The model under review builds one solid part; all positions refer to its coordinate system, in mm. A direction names the side the tool comes from. Coordinates: 2 decimals unless noted, no trailing zeros. Loops run counter-clockwise (first coordinate to the right, second up) from the corner with the lowest first, then second, coordinate; pieces in that order, holes last. Notation, with made-up numbers: M 26,-3.75 L 61,-3.75 A3 cw 61,0.25 Z; hole C 85,2 d6. An arc over 180 degrees is marked long. Return JSON: item names as keys, results as strings.
```python
from build123d import *

# Parameters (mm, degrees)
SKETCH_1_R          = 2
EXTRUDE_1_DEPTH     = 2
SKETCH_2_R          = 0.75
CUT_EXTRUDE_1_DEPTH = 102.941600929
FILLET_1_R          = 2
SKETCH_3_W          = 5.7
SKETCH_3_H          = 27.500414906
CUT_EXTRUDE_2_DEPTH = 102.941600929
FILLET_2_R          = 1


with BuildPart() as part:
    # 草图1 → 凸台-拉伸1 (new body)
    with BuildSketch(Plane(origin=(0, 0, 0), x_dir=(1, 0, 0), z_dir=(0, 1, 0))):
        Polygon((7.5, 100), (7.5, -7.5), (-7.5, -7.5), (-17.7, 12), (-17.7, 22), (-19.7, 22), (-19.7, 42), (-17.7, 42), (-17.7, 57), (-19.7, 57), (-19.7, 77), (-17.7, 77), (-17.7, 87), (-7.5, 100), align=None)
        with Locations(Location((0, 25, 0), (0, 0, 270))):
            Circle(SKETCH_1_R, mode=Mode.SUBTRACT)
        with Locations(Location((0, 0, 0), (0, 0, 270))):
            Circle(SKETCH_1_R, mode=Mode.SUBTRACT)
        with Locations(Location((0, 72, 0), (0, 0, 270))):
            Circle(SKETCH_1_R, mode=Mode.SUBTRACT)
        with Locations(Location((0, 95, 0), (0, 0, 270))):
            Circle(SKETCH_1_R, mode=Mode.SUBTRACT)
    extrude(amount=EXTRUDE_1_DEPTH)

    # 草图2 → 切除-拉伸1 (cut, through all)
    with BuildSketch(Plane(origin=(0, 2, 0), x_dir=(1, 0, 0), z_dir=(0, 1, 0))):
        with Locations((-17.7, 77.75)):
            Circle(SKETCH_2_R)
        with Locations((-17.7, 56.25)):
            Circle(SKETCH_2_R)
        with Locations((-17.7, 42.75)):
            Circle(SKETCH_2_R)
        with Locations((-17.7, 21.25)):
            Circle(SKETCH_2_R)
    extrude(amount=-CUT_EXTRUDE_1_DEPTH, mode=Mode.SUBTRACT)

    # 圆角1
    fillet_1_edges = [part.edges().sort_by_distance(p)[0] for p in [
        (-17.7, 1, -87),
        (-7.5, 1, -100),
        (7.5, 1, -100),
        (7.5, 1, 7.5),
        (-7.5, 1, 7.5),
        (-17.7, 1, -12),
    ]]
    fillet(fillet_1_edges, radius=FILLET_1_R)

    # 草图3 → 切除-拉伸2 (cut, through all)
    with BuildSketch(Plane(origin=(0, 2, 0), x_dir=(1, 0, 0), z_dir=(0, 1, 0))):
        with BuildLine():
            Line((-4, 9), (-4, 16))
            ThreePointArc((-4, 16), (0, 20), (4, 16))
            Line((4, 16), (4, 9))
            ThreePointArc((4, 9), (0, 5), (-4, 9))
        make_face()
        with BuildLine():
            Line((4, 63), (4, 34))
            ThreePointArc((4, 34), (0, 30), (-4, 34))
            Line((-4, 34), (-4, 63))
            ThreePointArc((-4, 63), (0, 67), (4, 63))
        make_face()
        Polygon((-7.5, 92.710034389), (-13.2, 85.445328506), (-13.2, 65.209619483), (-7.5, 65.209619483), align=None)
        Polygon((-13.2, 13.105848495), (-7.5, 2.208789672), (-7.5, 29.709204577), (-13.2, 29.709204577), align=None)
        with Locations((-10.35, 47.45941203)):
            Rectangle(SKETCH_3_W, SKETCH_3_H)
    extrude(amount=-CUT_EXTRUDE_2_DEPTH, mode=Mode.SUBTRACT)

    # 圆角2
    fillet_2_edges = [part.edges().sort_by_distance(p)[0] for p in [
        (-7.5, 1, -92.710034389),
        (-7.5, 1, -65.209619483),
        (-13.2, 1, -65.209619483),
        (-13.2, 1, -85.445328506),
        (-7.5, 1, -29.709204577),
        (-7.5, 1, -2.208789672),
        (-13.2, 1, -13.105848495),
        (-13.2, 1, -29.709204577),
        (-13.2, 1, -33.709204577),
        (-13.2, 1, -61.209619483),
        (-7.5, 1, -61.209619483),
        (-7.5, 1, -33.709204577),
        (-19.7, 1, -22),
        (-19.7, 1, -42),
        (-19.7, 1, -57),
        (-19.7, 1, -77),
    ]]
    fillet(fillet_2_edges, radius=FILLET_2_R)


solid = part.part
```
1. Add section A-A on x = 0. Give the boundary of the cut face in (y, z), plus the area to 3 significant figures.
Check values:
{"outline": "M 0,-100 L 2,-100 L 2,-97 L 0,-97 Z; M 0,-93 L 2,-93 L 2,-74 L 0,-74 Z; M 0,-70 L 2,-70 L 2,-67 L 0,-67 Z; M 0,-30 L 2,-30 L 2,-27 L 0,-27 Z; M 0,-23 L 2,-23 L 2,-20 L 0,-20 Z; M 0,-5 L 2,-5 L 2,-2 L 0,-2 Z; M 0,2 L 2,2 L 2,7.5 L 0,7.5 Z", "area": "79.0 mm²"}
2. To check wall thickness, follow line 1 (X direction, y = 1.25, z = -25); line 2 (Z direction, x = -18.5, y = 0.6); line 3 (X direction, y = 1.8, z = -73). State the ranges of each line that lie inside material, in increasing order.
Check values:
{"line 1": "-19.7 to -13.2, -7.5 to -2, 2 to 7.5", "line 2": "-77 to -57, -42 to -22", "line 3": "-19.7 to -13.2, -7.5 to -1.73, 1.73 to 7.5"}
3. Add section C-C on z = -64. Give the boundary of the cut face in (x, y).
Check values:
{"outline": "M -19.7,0 L -3.87,0 L -3.87,2 L -19.7,2 Z; M 3.87,0 L 7.5,0 L 7.5,2 L 3.87,2 Z"}
4. Add section D-D on y = 0.8. State how many separate pieces and enclosed holes the cut face has, plus the area to 3 significant figures.
Check values:
{"separate pieces": "1", "enclosed holes": "9", "area": "1,770 mm²"}
5. Insertion check: pin 1 Ø0.6 at (x, y) = (-10, 1.5) entering from -Z; pin 2 Ø0.6 at (x, y) = (-9.5, 0.5) entering from +Z; pin 3 Ø5 at (x, z) = (0, -72) entering from -Y; pin 4 Ø1 at (y, z) = (1, -47) entering from -X. Each pin has a flat end and moves straight along its axis. Give the tip position at first contact, or say it passes through.
Check values:
{"pin 1": "z = -97.2", "pin 2": "z = 4.25", "pin 3": "y = 0", "pin 4": "x = -17.7"}
6. The part is to be moulded in two halves that separate along Z. For faces 1 (the face through (0, 1, -20)), 2 (the face through (-6, 2, -47)), 3 (the face through (-7.5, 1, -17)), 4 (the face through (6.93, 1.01, -99.4)), say which applies: released by +Z, released by -Z, zero draft, split by the parting line, or undercut.
Check values:
{"face 1": "undercut", "face 2": "zero draft", "face 3": "undercut", "face 4": "released by -Z"}
7. Machinability: for faces 5 (the face through (-12.7, 0.99, -2.44)), 6 (the face through (-11.11, 1.01, -88.11)), which of the approach directions +Z, -Z, +X, -X, +Y, -Y give a long, thin tool a straight path to every point of the face, cutting with its end or side? Answer none if there is none.
Check values:
{"face 5": "+Z, -X, +Y, -Y", "face 6": "+Y, -Y"}
8. Add section B-B on z = -25. Give the boundary of the cut face in (x, y), plus the area to 3 significant figures.
Check values:
{"outline": "M -19.7,0 L -13.2,0 L -13.2,2 L -19.7,2 Z; M -7.5,0 L -2,0 L -2,2 L -7.5,2 Z; M 2,0 L 7.5,0 L 7.5,2 L 2,2 Z", "area": "35.0 mm²"}
